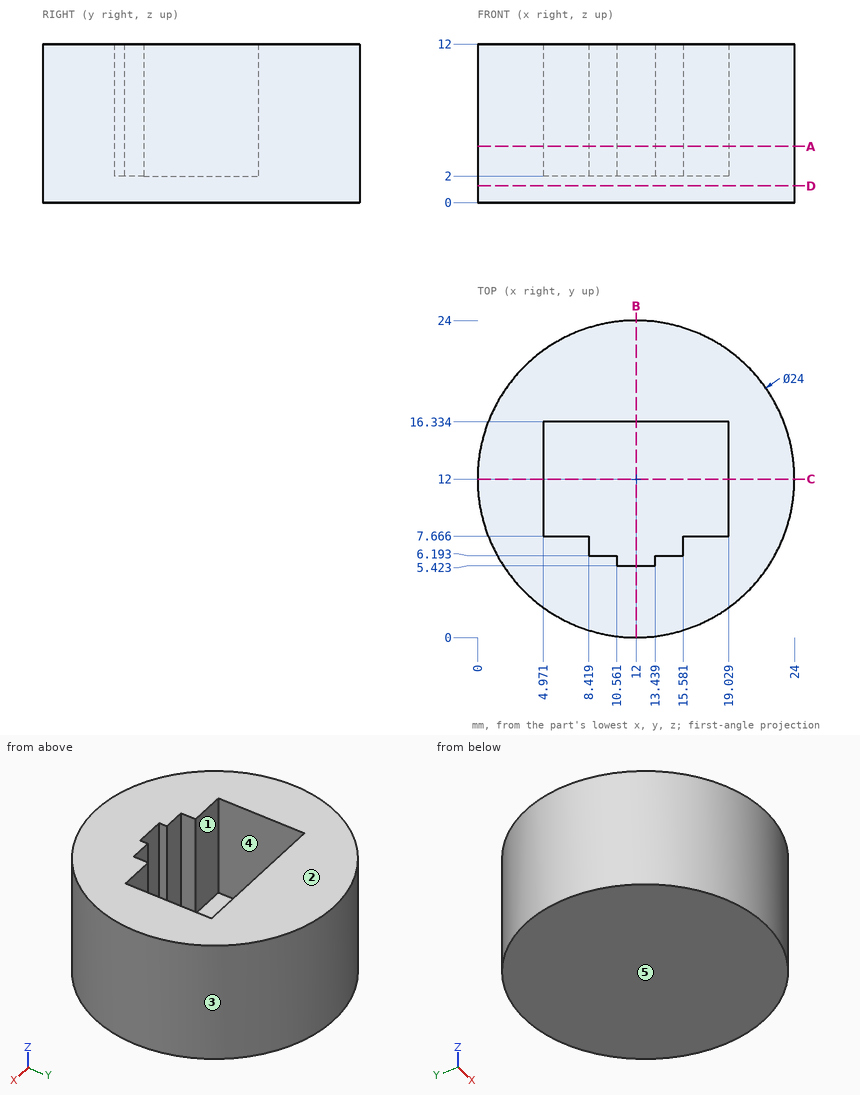
Drawing for the job (mm, zero at the part's lowest x, y, z). A direction names the side the tool comes from. Coordinates: 2 decimals unless noted, no trailing zeros. Write each loop counter-clockwise with the first axis right and the second up, starting at its lowest first coordinate (ties: lowest second). Pieces come first, ordered by that corner, then holes. Notation, with made-up numbers: (62.5, 9) - (103.5, 9) arc R19 ccw to (103.5, 15) - close; hole circle Ø3 at (-11, 17). An arc over 180 degrees is marked (long way). Write each question's results on one line, items separated by ' | '. Start each with the question number.
1) Mould opens along X. For the marked faces 3, 4 and 5 say: pulls with the +X half, pulls with the -X half, needs draft (parallel to the pull), parting line crosses it, or undercut.
2) 3-axis set-ups, long thin cutter, end or side, ignore diameter. For the marked faces 1 and 2: which of +Z, -Z, +X, -X, +Y, -Y reach the whole face in a straight line?
3) Cut at D-D (z = 1.25). Write the cut outline in (x, y).
4) Cut at B-B (x = 12). Write the cut outline in (y, z) (1 decimal).
5) Cut at C-C (y = 12). Write the cut outline in (x, z).
6) Probe line 1 along X through (y, z) = (14.5, 3); line 2 along X through (y, z) = (8, 8) (1 decimal); line 3 along Y through (x, z) = (9.75, 5.25) (1 decimal). List the from-to ranges inside material, lowest first. Write a range as from..to.
7) Flat gauge pins, fed straight in: P1, Ø1.1, axis at x = 15, z = 6, coming from the +Y side; P2, Ø0.6, axis at y = 5.5, z = 9, coming from the +X side (1 decimal); P3, Ø3.5, axis at x = 10.5, y = 12, coming from the +Z side. Where does each tip first touch, or does it go through?
8) Cut at A-A (z = 4.25). Write the cut outline in (x, y) (1 decimal).
Returned:
1) face 3: parting line crosses it | face 4: undercut | face 5: needs draft
2) face 1: +Z | face 2: +Z, +X, -X, +Y, -Y
3) outline: circle Ø24 at (12, 12)
4) outline: (0, 0) - (24, 0) - (24, 12) - (16.3, 12) - (16.3, 2) - (5.4, 2) - (5.4, 12) - (0, 12) - close
5) outline: (0, 0) - (24, 0) - (24, 12) - (19.03, 12) - (19.03, 2) - (4.97, 2) - (4.97, 12) - (0, 12) - close
6) line 1: 0.26..4.97, 19.03..23.74 | line 2: 0.7..5, 19..23.3 | line 3: 0.2..6.2, 16.3..23.8
7) P1: y = 23.75 | P2: x = 22.3 | P3: z = 2
8) outline: circle Ø24 at (12, 12); hole (5, 7.7) - (8.4, 7.7) - (8.4, 6.2) - (10.6, 6.2) - (10.6, 5.4) - (13.4, 5.4) - (13.4, 6.2) - (15.6, 6.2) - (15.6, 7.7) - (19, 7.7) - (19, 16.3) - (5, 16.3) - close
